Geometry: final body of the model. Coordinates: model frame, mm. Round coordinates to 2 decimals unless told otherwise and drop trailing zeros. Write item = value, one per line. Start each with the question number.
Item 1: Draft query along Y for faces 1 (the flat face through (760.643, 1006, 1347)), 2 (the flat face through (690, 932, 1335.724)). Return one class per face: pulls with the +Y half, pulls with the -Y half, needs draft (parallel to the pull), parting line crosses it, or undercut.
Item 2: Section A-A (x = 654). Count the separate pieces of the cut face and the enclosed holes in it, plus the area to 3 significant figures.
Item 3: First-contact query: pin 1 (11.5 mm diameter, centred on y = 922.5, z = 1342, fed in from -X); pin 2 (4 mm diameter, centred on x = 800.5, y = 863.5, fed in from +Z); pin 3 (5 mm diameter, centred on x = 648.5, z = 1347.5, fed in from +Y). Flat tips, straight axial feed; report the tip coordinate or a pass-through.
Item 4: Line query: line 1 (X direction, y = 870.5, z = 1345.5); line 2 (Y direction, x = 781.5, z = 1356.25); line 3 (Y direction, x = 662, z = 1355.25). Output: solid intervals per line, ascending. Write a range as from..to.
from build123d import *

# Parameters (mm, degrees)
SKETCH1_W           = 199.6
SKETCH1_H           = 199.6
BOSS_EXTRUDE1_DEPTH = 20
SKETCH2_W           = 226.2
SKETCH2_H           = 226.2
SKETCH2_W_2         = 220.2
SKETCH2_H_2         = 220.2
BOSS_EXTRUDE2_DEPTH = 5
SKETCH3_W           = 43.9
SKETCH3_H           = 43.9
CUT_EXTRUDE2_DEPTH  = 17
SKETCH4_W           = 226.2
SKETCH4_H           = 226.2
SKETCH4_R           = 1
SKETCH4_W_2         = 193.6
SKETCH4_H_2         = 193.6
BOSS_EXTRUDE3_DEPTH = 3
SKETCH5_W           = 20
SKETCH5_H           = 2.2
SKETCH5_W_2         = 2.2
SKETCH5_H_2         = 20
CUT_EXTRUDE3_DEPTH  = 1332.979018481
SKETCH6_W           = 232.2
SKETCH6_H           = 232.2
SKETCH6_W_2         = 226.2
SKETCH6_H_2         = 226.2
BOSS_EXTRUDE4_DEPTH = 8
BOSS_EXTRUDE5_DEPTH = 20
SKETCH8_R           = 4
CUT_EXTRUDE4_DEPTH  = 1337.192961728
FILLET1_R           = 2
FILLET2_R           = 1
SKETCH9_W           = 220.5
SKETCH9_H           = 220.5
SKETCH9_W_2         = 199.6
SKETCH9_H_2         = 199.6
CUT_EXTRUDE5_DEPTH  = 5
FILLET4_R           = 2


with BuildPart() as part:
    # Sketch1 → Boss-Extrude1 (new body)
    with BuildSketch(Plane.XY.offset(1355.724355858)):
        with Locations((713.742691035, 930.978191495)):
            Rectangle(SKETCH1_W, SKETCH1_H)
    extrude(amount=-BOSS_EXTRUDE1_DEPTH)

    # Sketch3 → Cut-Extrude2 (cut)
    with BuildSketch(Plane.XY.offset(1355.724355858)):
        with Locations((638.892691035, 906.028191495)):
            Rectangle(SKETCH3_W, SKETCH3_H)
        with Locations((638.892691035, 955.928191495)):
            Rectangle(SKETCH3_W, SKETCH3_H)
        with Locations((638.892691035, 856.128191495)):
            Rectangle(SKETCH3_W, SKETCH3_H)
        with Locations((788.592691035, 856.128191495)):
            Rectangle(SKETCH3_W, SKETCH3_H)
        with Locations((788.592691035, 1005.828191495)):
            Rectangle(SKETCH3_W, SKETCH3_H)
        with Locations((638.892691035, 1005.828191495)):
            Rectangle(SKETCH3_W, SKETCH3_H)
        with Locations((688.792691035, 1005.828191495)):
            Rectangle(SKETCH3_W, SKETCH3_H)
        with Locations((738.692691035, 1005.828191495)):
            Rectangle(SKETCH3_W, SKETCH3_H)
        with Locations((738.692691035, 955.928191495)):
            Rectangle(SKETCH3_W, SKETCH3_H)
        with Locations((688.792691035, 906.028191495)):
            Rectangle(SKETCH3_W, SKETCH3_H)
        with Locations((738.692691035, 906.028191495)):
            Rectangle(SKETCH3_W, SKETCH3_H)
        with Locations((688.792691035, 955.928191495)):
            Rectangle(SKETCH3_W, SKETCH3_H)
        with Locations((788.592691035, 955.928191495)):
            Rectangle(SKETCH3_W, SKETCH3_H)
        with Locations((738.692691035, 856.128191495)):
            Rectangle(SKETCH3_W, SKETCH3_H)
        with Locations((788.592691035, 906.028191495)):
            Rectangle(SKETCH3_W, SKETCH3_H)
        with Locations((688.792691035, 856.128191495)):
            Rectangle(SKETCH3_W, SKETCH3_H)
    extrude(amount=-CUT_EXTRUDE2_DEPTH, mode=Mode.SUBTRACT)



with BuildPart() as body_2:
    # Sketch2 → Boss-Extrude2 (new body)
    with BuildSketch(Plane.XY.offset(1355.724355858)):
        with Locations((713.742691035, 930.978191495)):
            Rectangle(SKETCH2_W, SKETCH2_H)
        with Locations((713.742691035, 930.978191495)):
            Rectangle(SKETCH2_W_2, SKETCH2_H_2, mode=Mode.SUBTRACT)
    extrude(amount=-BOSS_EXTRUDE2_DEPTH)


with BuildPart() as part_1:
    add(part.part)

    add(body_2.part)  # Boss-Extrude3 merges body 2
    # Sketch4 → Boss-Extrude3 (add)
    with BuildSketch(Plane.XY.offset(1355.724355858)):
        with Locations((713.742691035, 930.978191495)):
            Rectangle(SKETCH4_W, SKETCH4_H)
        with Locations((607.742691035, 1036.978191495)):
            Circle(SKETCH4_R, mode=Mode.SUBTRACT)
        with Locations((713.742691035, 1036.978191495)):
            Circle(SKETCH4_R, mode=Mode.SUBTRACT)
        with Locations((819.742691035, 1036.978191495)):
            Circle(SKETCH4_R, mode=Mode.SUBTRACT)
        with Locations((607.742691035, 930.978191495)):
            Circle(SKETCH4_R, mode=Mode.SUBTRACT)
        with Locations((607.742691035, 824.978191495)):
            Circle(SKETCH4_R, mode=Mode.SUBTRACT)
        with Locations((713.742691035, 824.978191495)):
            Circle(SKETCH4_R, mode=Mode.SUBTRACT)
        with Locations((819.742691035, 824.978191495)):
            Circle(SKETCH4_R, mode=Mode.SUBTRACT)
        with Locations((713.742691035, 930.978191495)):
            Rectangle(SKETCH4_W_2, SKETCH4_H_2, mode=Mode.SUBTRACT)
    extrude(amount=BOSS_EXTRUDE3_DEPTH)

    # Sketch5 → Cut-Extrude3 (cut, through all)
    with BuildSketch(Plane(origin=(0, 0, 1355.724355858), x_dir=(-1, 0, 0), z_dir=(0, 0, -1))):
        with Locations((-773.642691035, 1031.878191495)):
            Rectangle(SKETCH5_W, SKETCH5_H)
        with Locations((-773.642691035, 830.078191495)):
            Rectangle(SKETCH5_W, SKETCH5_H)
        with Locations((-653.842691035, 830.078191495)):
            Rectangle(SKETCH5_W, SKETCH5_H)
        with Locations((-653.842691035, 1031.878191495)):
            Rectangle(SKETCH5_W, SKETCH5_H)
        with Locations((-814.642691035, 871.078191495)):
            Rectangle(SKETCH5_W_2, SKETCH5_H_2)
        with Locations((-814.642691035, 990.878191495)):
            Rectangle(SKETCH5_W_2, SKETCH5_H_2)
        with Locations((-612.842691035, 990.878191495)):
            Rectangle(SKETCH5_W_2, SKETCH5_H_2)
        with Locations((-612.842691035, 871.078191495)):
            Rectangle(SKETCH5_W_2, SKETCH5_H_2)
    extrude(amount=-CUT_EXTRUDE3_DEPTH, mode=Mode.SUBTRACT)

    # Sketch6 → Boss-Extrude4 (add)
    with BuildSketch(Plane.XY.offset(1358.724355858)):
        with Locations((713.742691035, 930.978191495)):
            Rectangle(SKETCH6_W, SKETCH6_H)
        with Locations((713.742691035, 930.978191495)):
            Rectangle(SKETCH6_W_2, SKETCH6_H_2, mode=Mode.SUBTRACT)
    extrude(amount=-BOSS_EXTRUDE4_DEPTH)

    # Sketch7 → Boss-Extrude5 (add)
    with BuildSketch(Plane.XY.offset(1355.724355858)):
        Polygon((703.742691035, 930.978191495), (703.742691035, 940.978191495), (723.742691035, 940.978191495), (723.742691035, 920.978191495), (703.742691035, 920.978191495), align=None)
    extrude(amount=-BOSS_EXTRUDE5_DEPTH)

    # Sketch8 → Cut-Extrude4 (cut, through all)
    with BuildSketch(Plane.XY.offset(1355.724355858)):
        with Locations((713.742691035, 930.978191495)):
            Circle(SKETCH8_R)
    extrude(amount=-CUT_EXTRUDE4_DEPTH, mode=Mode.SUBTRACT)

    # Fillet1
    fillet1_edges = [part_1.edges().sort_by_distance(p)[0] for p in [
        (709.742691035, 930.978191495, 1355.724355858),
    ]]
    fillet(fillet1_edges, radius=FILLET1_R)

    # Fillet2
    fillet2_edges = [part_1.edges().sort_by_distance(p)[0] for p in [
        (703.742691035, 940.978191495, 1347.224355858),
        (723.742691035, 940.978191495, 1347.224355858),
        (723.742691035, 920.978191495, 1347.224355858),
        (703.742691035, 920.978191495, 1347.224355858),
    ]]
    fillet(fillet2_edges, radius=FILLET2_R)

    # Sketch9 → Cut-Extrude5 (cut)
    with BuildSketch(Plane(origin=(0, 0, 1350.724355858), x_dir=(-1, 0, 0), z_dir=(0, 0, -1))):
        with Locations((-713.742691035, 930.978191495)):
            Rectangle(SKETCH9_W, SKETCH9_H)
        with Locations((-713.742691035, 930.978191495)):
            Rectangle(SKETCH9_W_2, SKETCH9_H_2, mode=Mode.SUBTRACT)
    extrude(amount=-CUT_EXTRUDE5_DEPTH, mode=Mode.SUBTRACT)

    # Fillet4
    fillet4_edges = [part_1.edges().sort_by_distance(p)[0] for p in [
        (713.742691035, 820.728191495, 1350.724355858),
        (603.492691035, 930.978191495, 1350.724355858),
        (713.742691035, 1041.228191495, 1350.724355858),
        (823.992691035, 930.978191495, 1350.724355858),
    ]]
    fillet(fillet4_edges, radius=FILLET4_R)


solid = part_1.part
Taken from the geometry:
q1.face_1 = undercut
q1.face_2 = needs draft
q2.separate_pieces = 3
q2.enclosed_holes = 0
q2.area = 1,170 mm^2
q3.pin_1 = 613.94
q3.pin_2 = 1338.72
q3.pin_3 = 1030.78
q4.line_1 = 613.94..616.94, 660.84..666.84, 710.74..716.74, 760.64..766.64, 810.54..813.54
q4.line_2 = 814.88..828.98, 831.18..834.18, 1027.78..1030.78, 1032.98..1047.08
q4.line_3 = 814.88..820.73, 831.18..1030.78, 1041.23..1047.08
